Build history of the part. All positions in model axes, mm. Round coordinates to 2 decimals unless told otherwise and drop trailing zeros. Write each loop counter-clockwise with the first axis right and the second up, starting at its lowest first coordinate (ties: lowest second). Pieces come first, ordered by that corner, then holes.
1) Flat gauge pin, fed straight in: pin 1 (3.5 mm diameter, centred on x = 0.19, z = 23.28, fed in from -Y). Where does the tip first touch, or does it go through?
2) Wall check: probe 1 along Y at (x, z) = (10, 72); probe 2 along Y at (x, z) = (-8, 247) (3 decimals); probe 3 along X at (y, z) = (18, 255) (3 decimals). Give the ranges that are in metal, low to high.
3) Saw through at C-C (y = -0.5). State how many separate pieces and enclosed holes the cut face has, plus the area to 3 significant figures.
4) Saw through at B-B (z = 123.5). Write the cut outline in (x, y) (3 decimals), plus the area to 3 significant figures.
5) Saw through at A-A (x = 4.75). Write the cut outline in (y, z) (3 decimals), plus the area to 3 significant figures.
from build123d import *

# Parameters (mm, degrees)
SKETCH1_W           = 25.4
SKETCH1_H           = 50.8
SKETCH1_W_2         = 19.05
SKETCH1_H_2         = 44.45
BOSS_EXTRUDE1_DEPTH = 279.4
CUT_EXTRUDE1_DEPTH  = 282.699627263
FILLET1_R           = 3
MIRROR2_START       = -12.7
MIRROR2_DEPTH       = 3.175
SKETCH4_R           = 2
CUT_EXTRUDE2_DEPTH  = 285.264471927
SKETCH5_R           = 2
CUT_EXTRUDE3_DEPTH  = 10


# Read off the part's stored shape, not the designer's step: Mirror2
with BuildPart() as part:
    # Sketch1 → Boss-Extrude1 (new body)
    with BuildSketch(Plane.XY):
        Rectangle(SKETCH1_W, SKETCH1_H)
        Rectangle(SKETCH1_W_2, SKETCH1_H_2, mode=Mode.SUBTRACT)
    extrude(amount=BOSS_EXTRUDE1_DEPTH)

    # Sketch3 → Cut-Extrude1 (cut, through all)
    with BuildSketch(Plane(origin=(12.7, 0, 0), x_dir=(0, 0, -1), z_dir=(1, 0, 0))):
        Polygon((-271.4, -17.4), (-243.98156969, -17.4), (-271.4, 11.579844337), align=None)
        Polygon((-238.475, -11.579844337), (-211.05656969, 17.4), (-265.89343031, 17.4), align=None)
        Polygon((-232.96843031, -17.4), (-178.13156969, -17.4), (-205.55, 11.579844337), align=None)
        Polygon((-172.625, -11.579844337), (-145.20656969, 17.4), (-200.04343031, 17.4), align=None)
        Polygon((-139.7, -17.4), (-139.7, 11.579844337), (-167.11843031, -17.4), align=None)
        Polygon((-139.7, -17.4), (-112.28156969, -17.4), (-139.7, 11.579844337), align=None)
        Polygon((-79.35656969, 17.4), (-134.19343031, 17.4), (-106.775, -11.579844337), align=None)
        Polygon((-73.85, 11.579844337), (-101.26843031, -17.4), (-46.43156969, -17.4), align=None)
        Polygon((-13.50656969, 17.4), (-68.34343031, 17.4), (-40.925, -11.579844337), align=None)
        Polygon((-8, 11.579844337), (-35.41843031, -17.4), (-8, -17.4), align=None)
    extrude(amount=-CUT_EXTRUDE1_DEPTH, mode=Mode.SUBTRACT)

    # Fillet1
    fillet1_edges = [part.edges().sort_by_distance(p)[0] for p in [
        (11.1125, -17.4, 167.11843031),
        (11.1125, 11.579844337, 139.7),
        (11.1125, -17.4, 112.28156969),
        (11.1125, -11.579844337, 238.475),
        (11.1125, 17.4, 265.89343031),
        (11.1125, 17.4, 211.05656969),
        (11.1125, 11.579844337, 205.55),
        (11.1125, -17.4, 178.13156969),
        (11.1125, -17.4, 232.96843031),
        (11.1125, 17.4, 13.50656969),
        (11.1125, -11.579844337, 40.925),
        (11.1125, 17.4, 68.34343031),
        (11.1125, 11.579844337, 8),
        (11.1125, -17.4, 8),
        (11.1125, -17.4, 35.41843031),
        (11.1125, 17.4, 79.35656969),
        (11.1125, -11.579844337, 106.775),
        (11.1125, 17.4, 134.19343031),
        (11.1125, -17.4, 46.43156969),
        (11.1125, -17.4, 101.26843031),
        (11.1125, 11.579844337, 73.85),
        (11.1125, 11.579844337, 271.4),
        (11.1125, -17.4, 243.98156969),
        (11.1125, -17.4, 271.4),
        (11.1125, -11.579844337, 172.625),
        (11.1125, 17.4, 200.04343031),
        (11.1125, 17.4, 145.20656969),
    ]]
    fillet(fillet1_edges, radius=FILLET1_R)

    # Mirror2 outline → Mirror2 (add)
    with BuildSketch(Plane.YZ.offset(MIRROR2_START)):
        with BuildLine():
            Line((-17.4, 35.41843031), (-17.4, 28.450140974))
            ThreePointArc((-17.4, 28.450140974), (-15.586296427, 31.205626555), (-12.338199475, 30.629356107))
            Line((-12.338199475, 30.629356107), (-17.4, 35.41843031))
        make_face()
        with BuildLine():
            ThreePointArc((-14.4, 8), (-16.521320344, 8.878679656), (-17.4, 11))
            Line((-17.4, 11), (-17.4, 8))
            Line((-17.4, 8), (-14.4, 8))
        make_face()
        with BuildLine():
            Line((11.579844337, 8), (6.105685289, 13.179215133))
            ThreePointArc((6.105685289, 13.179215133), (6.831145553, 9.890415708), (4.043884765, 8))
            Line((4.043884765, 8), (11.579844337, 8))
        make_face()
        with BuildLine():
            ThreePointArc((17.4, 20.474859026), (15.586296427, 17.719373445), (12.338199475, 18.295643893))
            Line((12.338199475, 18.295643893), (17.4, 13.50656969))
            Line((17.4, 13.50656969), (17.4, 20.474859026))
        make_face()
        with BuildLine():
            Line((-11.579844337, 40.925), (-9.276528114, 38.745784867))
            ThreePointArc((-9.276528114, 38.745784867), (-10.214727589, 40.925), (-9.276528114, 43.104215133))
            Line((-9.276528114, 43.104215133), (-11.579844337, 40.925))
        make_face()
        with BuildLine():
            ThreePointArc((12.338199475, 63.554356107), (15.586296427, 64.130626555), (17.4, 61.375140974))
            Line((17.4, 61.375140974), (17.4, 68.34343031))
            Line((17.4, 68.34343031), (12.338199475, 63.554356107))
        make_face()
        with BuildLine():
            Line((-17.4, 101.26843031), (-17.4, 94.300140974))
            ThreePointArc((-17.4, 94.300140974), (-15.586296427, 97.055626555), (-12.338199475, 96.479356107))
            Line((-12.338199475, 96.479356107), (-17.4, 101.26843031))
        make_face()
        with BuildLine():
            ThreePointArc((-12.338199475, 51.220643893), (-15.586296427, 50.644373445), (-17.4, 53.399859026))
            Line((-17.4, 53.399859026), (-17.4, 46.43156969))
            Line((-17.4, 46.43156969), (-12.338199475, 51.220643893))
        make_face()
        with BuildLine():
            Line((11.579844337, 73.85), (9.276528114, 76.029215133))
            ThreePointArc((9.276528114, 76.029215133), (10.214727589, 73.85), (9.276528114, 71.670784867))
            Line((9.276528114, 71.670784867), (11.579844337, 73.85))
        make_face()
        with BuildLine():
            Line((-11.579844337, 106.775), (-9.276528114, 104.595784867))
            ThreePointArc((-9.276528114, 104.595784867), (-10.214727589, 106.775), (-9.276528114, 108.954215133))
            Line((-9.276528114, 108.954215133), (-11.579844337, 106.775))
        make_face()
        with BuildLine():
            ThreePointArc((17.4, 86.324859026), (15.586296427, 83.569373445), (12.338199475, 84.145643893))
            Line((12.338199475, 84.145643893), (17.4, 79.35656969))
            Line((17.4, 79.35656969), (17.4, 86.324859026))
        make_face()
        with BuildLine():
            Line((17.4, 134.19343031), (12.338199475, 129.404356107))
            ThreePointArc((12.338199475, 129.404356107), (15.586296427, 129.980626555), (17.4, 127.225140974))
            Line((17.4, 127.225140974), (17.4, 134.19343031))
        make_face()
        with BuildLine():
            Line((-17.4, 112.28156969), (-12.338199475, 117.070643893))
            ThreePointArc((-12.338199475, 117.070643893), (-15.586296427, 116.494373445), (-17.4, 119.249859026))
            Line((-17.4, 119.249859026), (-17.4, 112.28156969))
        make_face()
        with BuildLine():
            ThreePointArc((9.276528114, 141.879215133), (10.214727589, 139.7), (9.276528114, 137.520784867))
            Line((9.276528114, 137.520784867), (11.579844337, 139.7))
            Line((11.579844337, 139.7), (9.276528114, 141.879215133))
        make_face()
        with BuildLine():
            Line((-17.4, 167.11843031), (-17.4, 160.150140974))
            ThreePointArc((-17.4, 160.150140974), (-15.586296427, 162.905626555), (-12.338199475, 162.329356107))
            Line((-12.338199475, 162.329356107), (-17.4, 167.11843031))
        make_face()
        with BuildLine():
            Line((17.4, 145.20656969), (17.4, 152.174859026))
            ThreePointArc((17.4, 152.174859026), (15.586296427, 149.419373445), (12.338199475, 149.995643893))
            Line((12.338199475, 149.995643893), (17.4, 145.20656969))
        make_face()
        with BuildLine():
            ThreePointArc((12.338199475, 195.254356107), (15.586296427, 195.830626555), (17.4, 193.075140974))
            Line((17.4, 193.075140974), (17.4, 200.04343031))
            Line((17.4, 200.04343031), (12.338199475, 195.254356107))
        make_face()
        with BuildLine():
            Line((-11.579844337, 172.625), (-9.276528114, 170.445784867))
            ThreePointArc((-9.276528114, 170.445784867), (-10.214727589, 172.625), (-9.276528114, 174.804215133))
            Line((-9.276528114, 174.804215133), (-11.579844337, 172.625))
        make_face()
        with BuildLine():
            ThreePointArc((-12.338199475, 182.920643893), (-15.586296427, 182.344373445), (-17.4, 185.099859026))
            Line((-17.4, 185.099859026), (-17.4, 178.13156969))
            Line((-17.4, 178.13156969), (-12.338199475, 182.920643893))
        make_face()
        with BuildLine():
            Line((-17.4, 232.96843031), (-17.4, 226.000140974))
            ThreePointArc((-17.4, 226.000140974), (-15.586296427, 228.755626555), (-12.338199475, 228.179356107))
            Line((-12.338199475, 228.179356107), (-17.4, 232.96843031))
        make_face()
        with BuildLine():
            ThreePointArc((9.276528114, 207.729215133), (10.214727589, 205.55), (9.276528114, 203.370784867))
            Line((9.276528114, 203.370784867), (11.579844337, 205.55))
            Line((11.579844337, 205.55), (9.276528114, 207.729215133))
        make_face()
        with BuildLine():
            Line((-11.579844337, 238.475), (-9.276528114, 236.295784867))
            ThreePointArc((-9.276528114, 236.295784867), (-10.214727589, 238.475), (-9.276528114, 240.654215133))
            Line((-9.276528114, 240.654215133), (-11.579844337, 238.475))
        make_face()
        with BuildLine():
            ThreePointArc((17.4, 218.024859026), (15.586296427, 215.269373445), (12.338199475, 215.845643893))
            Line((12.338199475, 215.845643893), (17.4, 211.05656969))
            Line((17.4, 211.05656969), (17.4, 218.024859026))
        make_face()
        with BuildLine():
            Line((17.4, 265.89343031), (12.338199475, 261.104356107))
            ThreePointArc((12.338199475, 261.104356107), (15.586296427, 261.680626555), (17.4, 258.925140974))
            Line((17.4, 258.925140974), (17.4, 265.89343031))
        make_face()
        with BuildLine():
            ThreePointArc((-12.338199475, 248.770643893), (-15.586296427, 248.194373445), (-17.4, 250.949859026))
            Line((-17.4, 250.949859026), (-17.4, 243.98156969))
            Line((-17.4, 243.98156969), (-12.338199475, 248.770643893))
        make_face()
        with BuildLine():
            Line((-17.4, 271.4), (-17.4, 268.4))
            ThreePointArc((-17.4, 268.4), (-16.521320344, 270.521320344), (-14.4, 271.4))
            Line((-14.4, 271.4), (-17.4, 271.4))
        make_face()
        with BuildLine():
            ThreePointArc((4.043884765, 271.4), (6.831145553, 269.509584292), (6.105685289, 266.220784867))
            Line((6.105685289, 266.220784867), (11.579844337, 271.4))
            Line((11.579844337, 271.4), (4.043884765, 271.4))
        make_face()
    extrude(amount=MIRROR2_DEPTH)

    # Sketch4 → Cut-Extrude2 (cut, through all)
    with BuildSketch(Plane(origin=(0, 25.4, 0), x_dir=(1, 0, 0), z_dir=(0, 1, 0))):
        with Locations(Location((0.194187774, -256.116666667, 0), (0, 0, 270))):
            Circle(SKETCH4_R)
        with Locations(Location((0.194187774, -232.833333333, 0), (0, 0, 270))):
            Circle(SKETCH4_R)
        with Locations(Location((0.194187774, -23.283333333, 0), (0, 0, 270))):
            Circle(SKETCH4_R)
        with Locations(Location((0.194187774, -46.566666667, 0), (0, 0, 270))):
            Circle(SKETCH4_R)
    extrude(amount=-CUT_EXTRUDE2_DEPTH, mode=Mode.SUBTRACT)

    # Sketch5 → Cut-Extrude3 (cut)
    with BuildSketch(Plane.XZ.offset(25.4)):
        with Locations((0, 174.130820965)):
            Circle(SKETCH5_R)
        with Locations((0, 139.627653329)):
            Circle(SKETCH5_R)
        with Locations((0, 105.124485692)):
            Circle(SKETCH5_R)
    extrude(amount=-CUT_EXTRUDE3_DEPTH, mode=Mode.SUBTRACT)


solid = part.part
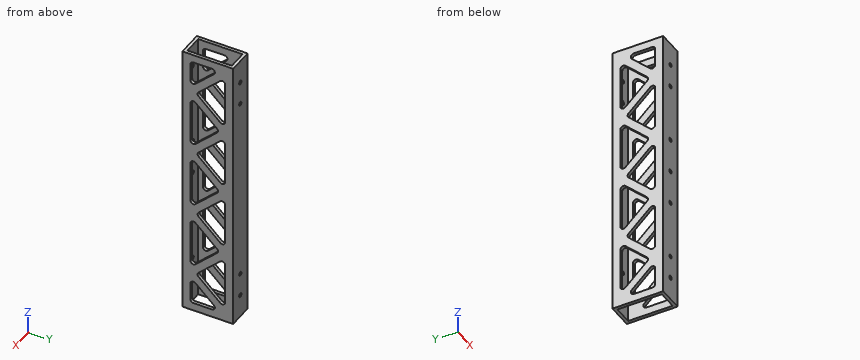
Evaluation:
1. pin 1: passes through
2. probe 1: y = -25.4 to -17.4, 9.58 to 25.4
2. probe 2: y = -25.4 to -22.225, 22.225 to 25.4
2. probe 3: x = -12.7 to -9.525, 9.525 to 12.7
3. separate pieces: 20
3. enclosed holes: 0
3. area: 661 mm2
4. outline: (-12.7, -25.4) - (12.7, -25.4) - (12.7, -17.4) - (9.525, -17.4) - (9.525, -22.225) - (-9.525, -22.225) - (-9.525, -17.4) - (-12.7, -17.4) - close; (-12.7, -5.543) - (-9.525, -5.543) - (-9.525, 6.098) - (-12.7, 6.098) - close; (-12.7, 17.4) - (-9.525, 17.4) - (-9.525, 22.225) - (9.525, 22.225) - (9.525, 17.4) - (12.7, 17.4) - (12.7, 25.4) - (-12.7, 25.4) - close; (9.525, -5.543) - (12.7, -5.543) - (12.7, 6.098) - (9.525, 6.098) - close
4. area: 296 mm2
5. outline: (-25.4, 0) - (-22.225, 0) - (-22.225, 279.4) - (-25.4, 279.4) - close; (22.225, 0) - (25.4, 0) - (25.4, 279.4) - (22.225, 279.4) - close
5. area: 1,770 mm2
